from build123d import *

# Parameters (mm, degrees)
SKETCH_1_R                       = 140
SKETCH_1_R_2                     = 40
EXTRUDE_1_DEPTH                  = 10
HOLE_WIZARD_20_0_20_1_AT_2_COUNT = 2
HOLE_WIZARD_20_0_20_1_AT_2_PITCH = 127.279220614
HOLE_WIZARD_20_0_20_1_AT_3_COUNT = 2
HOLE_WIZARD_20_0_20_1_AT_3_PITCH = 180
HOLE_WIZARD_20_0_20_1_AT_4_COUNT = 2
HOLE_WIZARD_20_0_20_1_AT_4_PITCH = 127.279220614


with BuildPart() as part:
    # Sketch 1 → Extrude 1 (new body)
    with BuildSketch(Plane(origin=(0, 0, 0), x_dir=(1, 0, 0), z_dir=(0, 1, 0))):
        with Locations(Location((0, 0, 0), (0, 0, 270))):
            Circle(SKETCH_1_R)
        with Locations(Location((0, 0, 0), (0, 0, 270))):
            Circle(SKETCH_1_R_2, mode=Mode.SUBTRACT)
    extrude(amount=EXTRUDE_1_DEPTH)

    # Sketch 3 → Hole Wizard 20.0 _20_ _1 (revolve, cut)
    with BuildSketch(Plane(origin=(0, 10, 90), x_dir=(0, 0, 1), z_dir=(1, 0, 0))):
        Polygon((0, 0), (0, 10), (10, 10), (10, 0.025), (10.025, 0), align=None)
    hole_wizard_20_0_20_1 = revolve(axis=Axis((0, 16.35, 90), (0, -1, 0)), mode=Mode.SUBTRACT)

    # Hole Wizard 20.0 _20_ _1 at 2: Hole Wizard 20.0 _20_ _1 ×2
    with Locations(*[Vector(0.7071067811865476, 0, -0.7071067811865476) * (i * HOLE_WIZARD_20_0_20_1_AT_2_PITCH) for i in range(1, HOLE_WIZARD_20_0_20_1_AT_2_COUNT)]):
        add(hole_wizard_20_0_20_1, mode=Mode.SUBTRACT)

    # Hole Wizard 20.0 _20_ _1 at 3: Hole Wizard 20.0 _20_ _1 ×2
    with Locations(*[(0, 0, -i * HOLE_WIZARD_20_0_20_1_AT_3_PITCH) for i in range(1, HOLE_WIZARD_20_0_20_1_AT_3_COUNT)]):
        add(hole_wizard_20_0_20_1, mode=Mode.SUBTRACT)

    # Hole Wizard 20.0 _20_ _1 at 4: Hole Wizard 20.0 _20_ _1 ×2
    with Locations(*[Vector(-0.7071067811865476, 0, -0.7071067811865476) * (i * HOLE_WIZARD_20_0_20_1_AT_4_PITCH) for i in range(1, HOLE_WIZARD_20_0_20_1_AT_4_COUNT)]):
        add(hole_wizard_20_0_20_1, mode=Mode.SUBTRACT)


solid = part.part
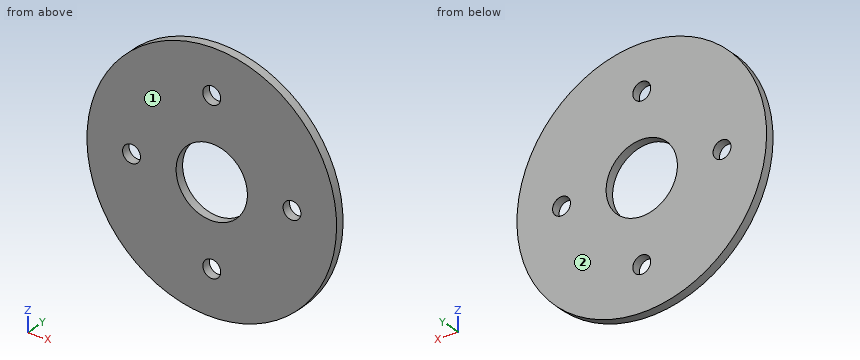
Work out the finished part from the listing and answer in its coordinate system (mm). Face numbers are marked on the shaded views. Round coordinates to 2 decimals unless told otherwise and drop trailing zeros. Loops run counter-clockwise (first coordinate to the right, second up) from the corner with the lowest first, then second, coordinate; pieces in that order, holes last. Notation, with made-up numbers: M 43.25,74 L 61.25,74 A20 cw 61.25,84 Z; hole C 78.5,-23.5 d2. An arc over 180 degrees is marked long. One line per question, with ' | ' between items. Start each with the question number.
(1) A cutting plane is placed at B-B on x = -16.5. Write down the section's boundary in (y, z).
(2) For a pull along Y with two mould halves and no side action, classify the marked faces 1 and 2 as released by +Y, released by -Y, zero draft, split by the parting line, or undercut.
(3) A cutting plane is placed at D-D on y = 8.25. Write down the section's boundary in (x, z), plus the area to 3 significant figures.
(4) A cutting plane is placed at C-C on z = -30. Write down the section's boundary in (x, y).
(5) A cutting plane is placed at A-A on z = 0. Write down the section's boundary in (x, y) (3 decimals).
(6) Find the intervals of material crossed by line 1 (X direction, y = 5.5, z = 0); line 2 (Z direction, x = 88, y = 3.5); line 3 (Z direction, x = 3, y = 8), in increasing order.
(7) Flat-ended cylindrical pins translate along their axes: pin 1 Ø2 at (x, y) = (17, 6.5) entering from +Z; pin 2 Ø18 at (x, z) = (-90, 0) entering from +Y; pin 3 Ø4 at (x, y) = (80, 7) entering from -Z; pin 4 Ø1.5 at (y, z) = (4, 93) entering from +X. Find the tip coordinate at first contact, or state that the pin passes through.
Geometry check:
1) outline: M 0,-139.02 L 10,-139.02 L 10,-36.44 L 0,-36.44 Z; M 0,36.44 L 10,36.44 L 10,139.02 L 0,139.02 Z
2) face 1: released by -Y | face 2: released by +Y
3) outline: C 0,0 d280; hole C -90,0 d20; hole C 0,0 d80; hole C 0,-90 d20; hole C 0,90 d20; hole C 90,0 d20 | area: 55,300 mm²
4) outline: M -136.75,0 L -26.46,0 L -26.46,10 L -136.75,10 Z; M 26.46,0 L 136.75,0 L 136.75,10 L 26.46,10 Z
5) outline: M -140,0 L -100,0 L -100,9.975 L -100.025,10 L -140,10 Z; M -80,0 L -40,0 L -40,10 L -79.975,10 L -80,9.975 Z; M 40,0 L 80,0 L 80,9.975 L 79.975,10 L 40,10 Z; M 100,0 L 140,0 L 140,10 L 100.025,10 L 100,9.975 Z
6) line 1: x = -140 to -100, -80 to -40, 40 to 80, 100 to 140 | line 2: z = -108.89 to -9.8, 9.8 to 108.89 | line 3: z = -139.97 to -99.54, -80.46 to -39.89, 39.89 to 80.46, 99.54 to 139.97
7) pin 1: stops at z = 139.08 | pin 2: passes through | pin 3: stops at z = -116.26 | pin 4: stops at x = 105.31
